Design review of the part built by this model. Coordinates are the model's own, in mm. Face numbers are marked on the shaded views. A direction names the side the tool comes from. Coordinates: 2 decimals unless noted, no trailing zeros. Order: outer loops, then holes, each group sorted by start corner. A loop starts at its lowest first (then second) coordinate and runs counter-clockwise, first axis right, second up. Notation, with made-up numbers: (-7, 31.5) - (46, 31.5) arc R29 ccw to (46, 54.5) - close; hole circle Ø8 at (29.5, 76). An arc over 180 degrees is marked (long way). Write each question's results on one line, items separated by ' | '. Start each with the question number.
```python
from build123d import *

# Parameters (mm, degrees)
SKETCH1_W               = 13.8
SKETCH1_H               = 8.8
BOSS_EXTRUDE1_DEPTH     = 3
SKETCH2_W               = 2
SKETCH2_H               = 35
BOSS_EXTRUDE2_DEPTH     = 3
SKETCH3_W               = 1.2
SKETCH3_H               = 6
BOSS_EXTRUDE3_DEPTH     = 7
FILLET3_R               = 10
SKETCH5_W               = 15
SKETCH5_H               = 13.8
BOSS_EXTRUDE4_DEPTH     = 4
SKETCH6_R               = 1.5
CUT_EXTRUDE4_DEPTH      = 38.968539608
BOSS_EXTRUDE5_DEPTH     = 2
CHAMFER2_SIZE           = 3
BOSS_EXTRUDE7_DEPTH     = 1.2
SKETCH12_W              = 15
SKETCH12_H              = 4
BOSS_EXTRUDE8_DEPTH     = 3
SKETCH13_W              = 15
SKETCH13_H              = 4
BOSS_EXTRUDE9_DEPTH     = 3
CUT_EXTRUDE7_DEPTH      = 43.28486727
CUT_EXTRUDE7_DEPTH_BACK = 43.28486727
CUT_EXTRUDE8_DEPTH      = 43.28486727
CUT_EXTRUDE8_DEPTH_BACK = 43.28486727
SKETCH15_W              = 0.807911756
SKETCH15_H              = 0.64
CUT_EXTRUDE9_DEPTH      = 41.244591358
CUT_EXTRUDE9_DEPTH_BACK = 41.244591358
SKETCH16_W              = 0.64
SKETCH16_H              = 0.6
CHAMFER3_SIZE           = 1


# Some blends are built 0.0001 mm under size
with BuildPart() as part:
    # Sketch1 → Boss-Extrude1 (new body)
    with BuildSketch(Plane(origin=(0, 0, 0), x_dir=(0, 0, -1), z_dir=(1, 0, 0))):
        Rectangle(SKETCH1_W, SKETCH1_H)
    extrude(amount=BOSS_EXTRUDE1_DEPTH)

    # Sketch2 → Boss-Extrude2 (add)
    with BuildSketch(Plane(origin=(3, 0, 0), x_dir=(0, 0, -1), z_dir=(1, 0, 0))):
        with Locations((0, -13.1)):
            Rectangle(SKETCH2_W, SKETCH2_H)
    extrude(amount=BOSS_EXTRUDE2_DEPTH)

    # Sketch3 → Boss-Extrude3 (add)
    with BuildSketch(Plane(origin=(6, 0, 0), x_dir=(0, 0, -1), z_dir=(1, 0, 0))):
        with Locations((0, -27.6)):
            Rectangle(SKETCH3_W, SKETCH3_H)
    extrude(amount=BOSS_EXTRUDE3_DEPTH)

    # Fillet3
    # the kernel refuses this fillet: 10 mm, written as the material it adds along each edge
    with BuildSketch(Plane(origin=(3, -4.4, 1), x_dir=(-1, 0, 0), z_dir=(0, 0, -1))) as fillet3_piece_1:
        with BuildLine():
            CenterArc((10, -7.141428429), FILLET3_R, 134.427004001, 45.572995999)
            Line((0, -7.141428429), (0, 0))
            Line((0, 0), (3, 0))
        make_face()
    extrude(amount=2)

    # Sketch5 → Boss-Extrude4 (add)
    with BuildSketch(Plane(origin=(0, 4.4, 0), x_dir=(1, 0, 0), z_dir=(0, 1, 0))):
        with Locations((-4.5, 0)):
            Rectangle(SKETCH5_W, SKETCH5_H)
    extrude(amount=BOSS_EXTRUDE4_DEPTH)

    # Sketch6 → Cut-Extrude4 (cut, through all)
    with BuildSketch(Plane.XZ.offset(-4.4)):
        with Locations(Location((-6, 3, 0), (0, 0, 270))):
            Circle(SKETCH6_R)
        with Locations(Location((-6, -3, 0), (0, 0, 270))):
            Circle(SKETCH6_R)
    extrude(amount=-CUT_EXTRUDE4_DEPTH, mode=Mode.SUBTRACT)

    # Sketch8 → Boss-Extrude5 (add)
    with BuildSketch(Plane(origin=(0, 0, -1), x_dir=(-1, 0, 0), z_dir=(0, 0, -1))):
        Polygon((-3, -18.758153574), (0, -4.4), (-3, -4.4), align=None)
    extrude(amount=-BOSS_EXTRUDE5_DEPTH)

    # Chamfer2
    chamfer2_edges = [part.edges().sort_by_distance(p)[0] for p in [
        (3, 4.4, 0),
    ]]
    chamfer(chamfer2_edges, length=CHAMFER2_SIZE - 0.0001)  # a hair under: the kernel refuses the full size

    # Sketch11 → Boss-Extrude7 (add)
    with BuildSketch(Plane(origin=(0, 0, -0.6), x_dir=(-1, 0, 0), z_dir=(0, 0, -1))):
        Polygon((-6, -24.6), (-13, -24.6), (-6, 1.742521041), align=None)
    extrude(amount=-BOSS_EXTRUDE7_DEPTH)

    # Sketch12 → Boss-Extrude8 (add)
    with BuildSketch(Plane(origin=(0, 0, -6.9), x_dir=(-1, 0, 0), z_dir=(0, 0, -1))):
        with Locations((4.5, 6.4)):
            Rectangle(SKETCH12_W, SKETCH12_H)
    extrude(amount=BOSS_EXTRUDE8_DEPTH)

    # Sketch13 → Boss-Extrude9 (add)
    with BuildSketch(Plane.XY.offset(6.9)):
        with Locations((-4.5, 6.4)):
            Rectangle(SKETCH13_W, SKETCH13_H)
    extrude(amount=BOSS_EXTRUDE9_DEPTH)

    # Sketch14 → Cut-Extrude7 (cut, two sides: drawn at the far end of the back side and taken through both)
    with BuildSketch(Plane(origin=(0, 8.4, 0), x_dir=(1, 0, 0), z_dir=(0, 1, 0)).offset(-CUT_EXTRUDE7_DEPTH_BACK)):
        with BuildLine():
            Line((-7.5, 7), (-7.5, -7))
            ThreePointArc((-7.5, -7), (-6, -8.5), (-4.5, -7))
            Line((-4.5, -7), (-4.5, 7))
            ThreePointArc((-4.5, 7), (-6, 8.5), (-7.5, 7))
        make_face()
    extrude(amount=CUT_EXTRUDE7_DEPTH + CUT_EXTRUDE7_DEPTH_BACK, mode=Mode.SUBTRACT)

    # Sketch15 → Cut-Extrude8 (cut, two sides: drawn at the far end of the back side and taken through both)
    with BuildSketch(Plane.XZ.offset(30.6).offset(-CUT_EXTRUDE8_DEPTH_BACK)):
        with Locations((12.596044122, 0)):
            Rectangle(SKETCH15_W, SKETCH15_H)
    extrude(amount=CUT_EXTRUDE8_DEPTH + CUT_EXTRUDE8_DEPTH_BACK, mode=Mode.SUBTRACT)

    # Sketch16 → Cut-Extrude9 (cut, two sides: drawn at the far end of the back side and taken through both)
    with BuildSketch(Plane(origin=(12.192088244, 0, 0), x_dir=(0, 0, -1), z_dir=(1, 0, 0)).offset(-CUT_EXTRUDE9_DEPTH_BACK)):
        with Locations((0, -30.3)):
            Rectangle(SKETCH16_W, SKETCH16_H)
    extrude(amount=CUT_EXTRUDE9_DEPTH + CUT_EXTRUDE9_DEPTH_BACK, mode=Mode.SUBTRACT)

    # Chamfer3
    chamfer3_edges = [part.edges().sort_by_distance(p)[0] for p in [
        (12.192088244, -30, 0),
    ]]
    chamfer(chamfer3_edges, length=CHAMFER3_SIZE)


solid = part.part
```
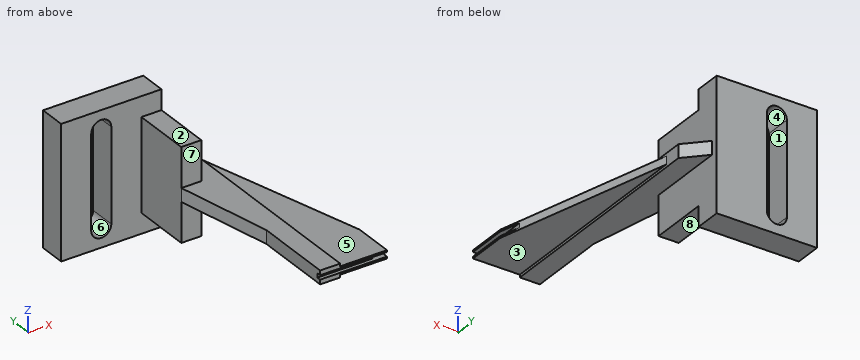
(1) Mouldability with a two-part tool opening along Z and no side actions: class the marked faces 1, 2, 3 and 4 as +Z half, -Z half, draft (parallel to the pull), parting line (faces both ways), or undercut.
(2) Tool access review of the marked faces 5, 6, 7 and 8: name each direction out of +Z, -Z, +X, -X, +Y, -Y from which nothing blocks a thin tool from reaching the whole face with its end or side.
(3) Take a section at C-C (y = -25.5). State the section outline as (x, z) points.
(4) Clearance check with flat-ended pins moving along their axes: pin 1 (4.5 mm diameter, centred on x = 8.5, y = -28, fed in from -Z); pin 2 (6 mm diameter, centred on x = 8.5, y = -18, fed in from -Z); pin 3 (3 mm diameter, centred on x = 3, y = -7.5, fed in from +Z). State where each tip first meets the part, or that it passes through.
(5) Take a section at B-B (x = -6). State the section outline as (y, z) points.
(6) To check wall thickness, follow line 1 along X through (y, z) = (6, 1.5); line 2 along Y through (x, z) = (-8, -0.25); line 3 along Z through (x, y) = (9, -25). State the ranges of each line that lie inside material, in increasing order. Write a range as [from, to].
(7) Take a section at A-A (z = 2.25). State the section outline as (x, y) points.
(8) Take a section at D-D (x = 4.75). State the section outline as (y, z) points, plus the area to 3 significant figures.
Worked out:
1) face 1: undercut | face 2: +Z half | face 3: -Z half | face 4: undercut
2) face 5: +Z, +X, +Y, -Y | face 6: +Y, -Y | face 7: +Z, +X, -X, -Y | face 8: -Z, +X, -X, -Y
3) outline: (3, -1) - (6, -1) - (6, -0.6) - (13, -0.6) - (13, -0.32) - (12.19, -0.32) - (12.19, 0.32) - (13, 0.32) - (13, 0.6) - (6, 0.6) - (6, 1) - (3, 1) - close
4) pin 1: z = -0.6 | pin 2: z = -1 | pin 3: z = 1
5) outline: (4.4, -9.9) - (8.4, -9.9) - (8.4, -8.5) - (4.4, -8.5) - close; (4.4, 8.5) - (8.4, 8.5) - (8.4, 9.9) - (4.4, 9.9) - close
6) line 1: [-12, -7.5], [-4.5, 3] | line 2: [4.4, 8.4] | line 3: [-0.6, 0.6]
7) outline: (-12, 4.4) - (-7.5, 4.4) - (-7.5, 8.4) - (-12, 8.4) - close; (-4.5, 4.4) - (0, 4.4) - (0, -4.4) - (3, -4.4) - (3, 8.4) - (-4.5, 8.4) - close
8) outline: (-30.6, -1) - (5.65, -1) - (5.65, 1) - (-30.6, 1) - (-30.6, 0.32) - (-30, 0.32) - (-30, -0.32) - (-30.6, -0.32) - close | area: 72.1 mm^2
